from build123d import *

# Parameters (mm, degrees)
SKETCH3_W         = 0.53
SKETCH3_H         = 2.14
SKETCH4_W         = 0.265
SKETCH4_H         = 0.265
CIRPATTERN1_COUNT = 2
CIRPATTERN1_ANGLE = 90


with BuildPart() as part:
    # BodySke → Base-Revolve (revolve)
    with BuildSketch(Plane.XY):
        Polygon((0, 0), (0, 1.9), (0.3, 1.9), (1.2, 1), (10, 1), (10, 0), align=None)
    revolve(axis=Axis((-6.35, 0, 0), (1, 0, 0)))

    # Sketch3 → Cross section 0
    with BuildSketch(Plane.ZY):
        Rectangle(SKETCH3_W, SKETCH3_H)
    # Sketch4 → Cross section 1
    with BuildSketch(Plane.ZY.offset(-1.54)):
        Rectangle(SKETCH4_W, SKETCH4_H)
    cross = loft(mode=Mode.SUBTRACT)

    # CirPattern1: Cross ×2 about axis
    cirpattern1_axis = Axis((0, 0, 0), (1, 0, 0))
    for i in range(1, CIRPATTERN1_COUNT):
        add(cross.rotate(cirpattern1_axis, i * CIRPATTERN1_ANGLE / (CIRPATTERN1_COUNT - 1)), mode=Mode.SUBTRACT)


solid = part.part
Read the model definition and answer for the solid it produces. Units are mm, in the model's axes. A direction names the side the tool comes from. Give positions to 0.01 mm unless a question says otherwise; leave off trailing zeros. Write each loop counter-clockwise with the first axis right and the second up, starting at its lowest first coordinate (ties: lowest second). Pieces come first, ordered by that corner, then holes. Notation, with made-up numbers: M 16.5,-22 L 44.5,-22 A15 ccw 44.5,-15 Z; hole C 14,69.5 d2. An arc over 180 degrees is marked long. One line per item, written item: value. Start each with the question number.
(1) A tool of negligible diameter and unlimited length cuts with its end or side. For faces 1 (the flat face through (0, 0.45, 0.45)), 2 (the cylindrical face through (6, 0, -1)), from which of +Z, -Z, +X, -X, +Y, -Y can it reach the whole face along a straight path? Write none if from no direction.
(2) Find the intervals of material crossed by line 1 (X direction, y = -0.05, z = 0); line 2 (X direction, y = 1.25, z = 0.7); line 3 (Z direction, x = 6.25, y = 0.4), in increasing order.
(3) Find section A-A (x = 3.5). Determine the outline of the cut face in (y, z).
(4) Flat-ended cylindrical pins translate along their axes: pin 1 Ø1 at (x, y) = (9, 0) entering from -Z; pin 2 Ø2 at (y, z) = (-0.5, -1.5) entering from -X. Find the tip coordinate at first contact, or state that the pin passes through.
Results below:
1. face 1: +Z, -Z, -X, +Y, -Y
1. face 2: +X
2. line 1: x = 1.54 to 10
2. line 2: x = 0 to 0.77
2. line 3: z = -0.92 to 0.92
3. outline: C 0,0 d2
4. pin 1: stops at z = -1
4. pin 2: stops at x = 0
